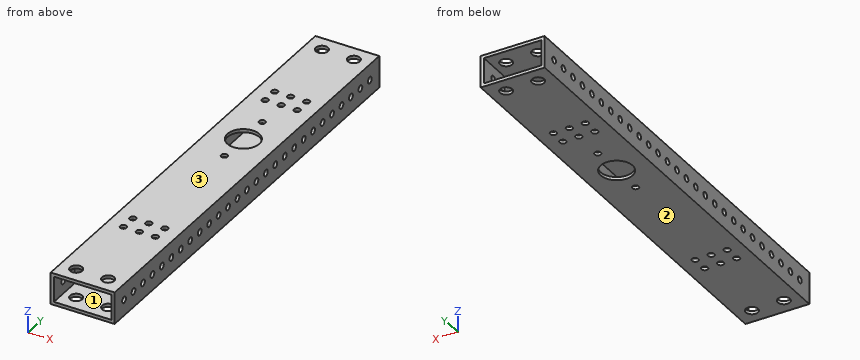
from build123d import *

# Parameters (mm, degrees)
SKETCH1_W           = 50.8
SKETCH1_H           = 25.4
SKETCH1_W_2         = 45.72
SKETCH1_H_2         = 20.32
BOSS_EXTRUDE1_DEPTH = 355.6
SKETCH2_R           = 2.54
CUT_EXTRUDE2_DEPTH  = 355.6
SKETCH3_R           = 4.826
SKETCH3_R_2         = 2.54
SKETCH3_R_3         = 12.7
CUT_EXTRUDE3_DEPTH  = 355.6


with BuildPart() as part:
    # Sketch1 → Boss-Extrude1 (new body)
    with BuildSketch(Plane(origin=(0, 0, 0), x_dir=(1, 0, 0), z_dir=(0, 1, 0))):
        with Locations((-23.021504389, 9.552608696)):
            Rectangle(SKETCH1_W, SKETCH1_H)
        with Locations((-23.021504389, 9.552608696)):
            Rectangle(SKETCH1_W_2, SKETCH1_H_2, mode=Mode.SUBTRACT)
    extrude(amount=BOSS_EXTRUDE1_DEPTH)

    # Sketch2 → Cut-Extrude2 (cut)
    with BuildSketch(Plane(origin=(2.378495611, 0, 0), x_dir=(0, 0, -1), z_dir=(1, 0, 0))):
        with Locations((9.552608696, 342.9)):
            Circle(SKETCH2_R)
        with Locations((9.552608696, 330.2)):
            Circle(SKETCH2_R)
        with Locations((9.552608696, 317.5)):
            Circle(SKETCH2_R)
        with Locations((9.552608696, 304.8)):
            Circle(SKETCH2_R)
        with Locations((9.552608696, 292.1)):
            Circle(SKETCH2_R)
        with Locations((9.552608696, 279.4)):
            Circle(SKETCH2_R)
        with Locations((9.552608696, 266.7)):
            Circle(SKETCH2_R)
        with Locations((9.552608696, 254)):
            Circle(SKETCH2_R)
        with Locations((9.552608696, 241.3)):
            Circle(SKETCH2_R)
        with Locations((9.552608696, 228.6)):
            Circle(SKETCH2_R)
        with Locations((9.552608696, 215.9)):
            Circle(SKETCH2_R)
        with Locations((9.552608696, 203.2)):
            Circle(SKETCH2_R)
        with Locations((9.552608696, 190.5)):
            Circle(SKETCH2_R)
        with Locations((9.552608696, 177.8)):
            Circle(SKETCH2_R)
        with Locations((9.552608696, 165.1)):
            Circle(SKETCH2_R)
        with Locations((9.552608696, 152.4)):
            Circle(SKETCH2_R)
        with Locations((9.552608696, 139.7)):
            Circle(SKETCH2_R)
        with Locations((9.552608696, 127)):
            Circle(SKETCH2_R)
        with Locations((9.552608696, 114.3)):
            Circle(SKETCH2_R)
        with Locations((9.552608696, 101.6)):
            Circle(SKETCH2_R)
        with Locations((9.552608696, 88.9)):
            Circle(SKETCH2_R)
        with Locations((9.552608696, 76.2)):
            Circle(SKETCH2_R)
        with Locations((9.552608696, 63.5)):
            Circle(SKETCH2_R)
        with Locations((9.552608696, 50.8)):
            Circle(SKETCH2_R)
        with Locations((9.552608696, 38.1)):
            Circle(SKETCH2_R)
        with Locations((9.552608696, 25.4)):
            Circle(SKETCH2_R)
        with Locations((9.552608696, 12.7)):
            Circle(SKETCH2_R)
    extrude(amount=-CUT_EXTRUDE2_DEPTH, mode=Mode.SUBTRACT)

    # Sketch3 → Cut-Extrude3 (cut)
    with BuildSketch(Plane(origin=(0, 0, -22.252608696), x_dir=(-1, 0, 0), z_dir=(0, 0, -1))):
        with Locations((10.321504389, 342.9)):
            Circle(SKETCH3_R)
        with Locations((35.721504389, 342.9)):
            Circle(SKETCH3_R)
        with Locations((10.321504389, 279.4)):
            Circle(SKETCH3_R_2)
        with Locations((23.021504389, 279.4)):
            Circle(SKETCH3_R_2)
        with Locations((35.721504389, 279.4)):
            Circle(SKETCH3_R_2)
        with Locations((10.321504389, 266.7)):
            Circle(SKETCH3_R_2)
        with Locations((23.021504389, 266.7)):
            Circle(SKETCH3_R_2)
        with Locations((35.721504389, 266.7)):
            Circle(SKETCH3_R_2)
        with Locations((23.021504389, 241.3)):
            Circle(SKETCH3_R_2)
        with Locations((23.021504389, 215.9)):
            Circle(SKETCH3_R_3)
        with Locations((23.021504389, 190.5)):
            Circle(SKETCH3_R_2)
        with Locations((35.721504389, 88.9)):
            Circle(SKETCH3_R_2)
        with Locations((23.021504389, 88.9)):
            Circle(SKETCH3_R_2)
        with Locations((10.321504389, 88.9)):
            Circle(SKETCH3_R_2)
        with Locations((10.321504389, 76.2)):
            Circle(SKETCH3_R_2)
        with Locations((23.021504389, 76.2)):
            Circle(SKETCH3_R_2)
        with Locations((35.721504389, 76.2)):
            Circle(SKETCH3_R_2)
        with Locations((35.721504389, 12.7)):
            Circle(SKETCH3_R)
        with Locations((10.321504389, 12.7)):
            Circle(SKETCH3_R)
    extrude(amount=-CUT_EXTRUDE3_DEPTH, mode=Mode.SUBTRACT)


solid = part.part
Geometry check sheet. Reference: the model listing, model coordinates, mm. Face numbers are marked on the shaded views. Round coordinates to 2 decimals unless told otherwise and drop trailing zeros. Order: outer loops, then holes, each group sorted by start corner. A loop starts at its lowest first (then second) coordinate and runs counter-clockwise, first axis right, second up. Notation, with made-up numbers: M 75.25,15.25 L 91.25,15.25 A30 ccw 91.25,46.25 Z; hole C 19.5,75 d9. An arc over 180 degrees is marked long. Answer in a Markdown table with one row per item.
(1) Sectioned sample at A-A, the plane z = -16. Record the cut outline in (x, y), and give its area (3 significant figures).
Responses:
| item | result |
|---|---|
| outline | M -48.42,0 L -45.88,0 L -45.88,355.6 L -48.42,355.6 Z; M -0.16,0 L 2.38,0 L 2.38,355.6 L -0.16,355.6 Z |
| area | 1,810 mm² |
(2) Draft check along Z on the marked faces 1, 2 and 3. Enter one of: released by +Z, released by -Z, zero draft, split by the parting line, or undercut.
Responses:
| item | result |
|---|---|
| face 1 | undercut |
| face 2 | released by -Z |
| face 3 | released by +Z |
(3) Scan lines: probe 1 along Z at (x, y) = (-40.5, 124); probe 2 along X at (y, z) = (210, 0.25); probe 3 along X at (y, z) = (190.5, 2.2). Record each from-to range of solid material in increasing order. Write a range as from..to.
Responses:
| item | result |
|---|---|
| probe 1 | z = -22.25..-19.71, 0.61..3.15 |
| probe 2 | x = -48.42..-45.88, -0.16..2.38 |
| probe 3 | x = -48.42..-25.56, -20.48..2.38 |
(4) Go/stop test with a flat-tipped pin: P1, Ø4, axis at y = 139.7, z = -9.55, coming from the +X side. Record where the tip stops, or that it passes through.
Responses:
| item | result |
|---|---|
| P1 | passes through |
